Build history of the part. All positions in model axes, mm. A direction names the side the tool comes from. Coordinates: 2 decimals unless noted, no trailing zeros. Loops run counter-clockwise (first coordinate to the right, second up) from the corner with the lowest first, then second, coordinate; pieces in that order, holes last. Notation, with made-up numbers: (51.5, 77) -> (103.5, 77) arc R13 cw to (103.5, 94) -> close; hole circle Ø3 at (41, -34). An arc over 180 degrees is marked (long way). One line per item, written item: value. Start each with the question number.
```python
from build123d import *

# Parameters (mm, degrees)
SKETCH1_W           = 20
SKETCH1_H           = 10
BOSS_EXTRUDE1_DEPTH = 1.3
SKETCH2_W           = 1.4
SKETCH2_H           = 6
BOSS_EXTRUDE2_DEPTH = 1.3
SKETCH3_W           = 20
SKETCH3_H           = 4
BOSS_EXTRUDE3_DEPTH = 1.3


with BuildPart() as part:
    # Sketch1 → Boss-Extrude1 (new body)
    with BuildSketch(Plane(origin=(0, 0, 0), x_dir=(1, 0, 0), z_dir=(0, 1, 0))):
        Rectangle(SKETCH1_W, SKETCH1_H)
    extrude(amount=BOSS_EXTRUDE1_DEPTH)

    # Sketch2 → Boss-Extrude2 (add)
    with BuildSketch(Plane(origin=(0, 1.3, 0), x_dir=(1, 0, 0), z_dir=(0, 1, 0))):
        with Locations((-10.7, 0)):
            Rectangle(SKETCH2_W, SKETCH2_H)
        with Locations((10.7, 0)):
            Rectangle(SKETCH2_W, SKETCH2_H)
    extrude(amount=-BOSS_EXTRUDE2_DEPTH)

    # Sketch3 → Boss-Extrude3 (add)
    with BuildSketch(Plane(origin=(0, 1.3, 0), x_dir=(1, 0, 0), z_dir=(0, 1, 0))):
        with Locations((0, 7)):
            Rectangle(SKETCH3_W, SKETCH3_H)
    extrude(amount=-BOSS_EXTRUDE3_DEPTH)


solid = part.part
```
Item 1: Band-saw the part on B-B, the plane z = 3.5. List the corners of the cut face in (x, y), and give its area (3 significant figures).
Item 2: Tool access for faces 1 (the face through (11, 1, -3)), 2 (the face through (-11, 1, 3)), 3 (the face through (-11, 1, -3)), 4 (the face through (10, 1, 4)): list every direction of +Z, -Z, +X, -X, +Y, -Y with a clear straight run to the whole face (end or side of a thin tool).
Item 3: Drop flat-ended pins along their axis: pin 1 Ø0.6 at (x, y) = (10.5, 1) entering from -Z; pin 2 Ø0.6 at (x, y) = (-10.5, 1) entering from +Z; pin 3 Ø1 at (x, z) = (-7, 2.5) entering from -Y. Give the stop position or say it passes through.
Item 4: Probe probe 1 along X at (y, z) = (1.05, -6). List the from-to ranges inside material, lowest first.
Item 5: Band-saw the part on A-A, the plane y = 0.25. List the corners of the cut face in (x, z).
Worked out:
1. outline: (-10, 0) -> (10, 0) -> (10, 1.3) -> (-10, 1.3) -> close
1. area: 26.0 mm²
2. face 1: -Z, +X, +Y, -Y
2. face 2: +Z, -X, +Y, -Y
2. face 3: -Z, -X, +Y, -Y
2. face 4: +Z, +X, +Y, -Y
3. pin 1: stops at z = -3
3. pin 2: stops at z = 3
3. pin 3: stops at y = 0
4. probe 1: x = -10 to 10
5. outline: (-11.4, -3) -> (-10, -3) -> (-10, -9) -> (10, -9) -> (10, -3) -> (11.4, -3) -> (11.4, 3) -> (10, 3) -> (10, 5) -> (-10, 5) -> (-10, 3) -> (-11.4, 3) -> close
